from build123d import *

# Parameters (mm, degrees)
F0_R     = 10
F1_DEPTH = 25
F4_R     = 4
F5_DEPTH = 25


with BuildPart() as f1:
    # F0 (on Right) → F1 (new body)
    with BuildSketch(Plane.YZ):
        Circle(F0_R)
    extrude(amount=F1_DEPTH)


with BuildPart() as f2_1:
    # F2: copy of F1
    add(f1.part)

    # F4 (on face) → F5 (cut, through all)
    with BuildSketch(Plane.YZ.offset(25)):
        Circle(F4_R)
    extrude(amount=-F5_DEPTH, mode=Mode.SUBTRACT)


solid = f2_1.part
Part model, mm, in its own coordinate system. Round coordinates to 2 decimals unless told otherwise and drop trailing zeros. Write each loop counter-clockwise with the first axis right and the second up, starting at its lowest first coordinate (ties: lowest second). Pieces come first, ordered by that corner, then holes. Notation, with made-up numbers: M 20.25,74.25 L 61.25,74.25 A31 cw 61.25,100.25 Z; hole C 9,-17 d10. An arc over 180 degrees is marked long. Return JSON: item names as keys, results as strings. Group by question number.
(1) Saw through at D-D on x = 18. Write the cut outline in (y, z), then the cut area to 3 significant figures.
(2) Two-plate mould, pull along Z, no slides. Class faces 1 (the face through (0, -0.1, -4.3)), 2 (the face through (12.675, -0.867, -3.905)), 3 (the face through (12.32, -2.17, -9.76)): +Z half, -Z half, draft (parallel to the pull), parting line (faces both ways), or undercut.
(3) Drill centre lines: probe 1 along Z at (x, y) = (13.25, 0); probe 2 along Y at (x, z) = (22.25, 1.25); probe 3 along Z at (x, y) = (18.75, -1). Where is each one in solid material? Low to high.
(4) Pin check, flat tips, straight feed: pin 1 Ø7 at (y, z) = (0, 0) entering from +X; pin 2 Ø10 at (x, y) = (21, 6.5) entering from -Z; pin 3 Ø6 at (x, y) = (15, 8) entering from -Z. Stop position of each tip, or through.
(5) Saw through at A-A on z = 0. Write the cut outline in (x, y).
(6) Saw through at C-C on y = -8. Write the cut outline in (x, z), then the cut area to 3 significant figures.
Returned:
{
 "1": {"outline": "C 0,0 d20; hole C 0,0 d8", "area": "264 mm²"},
 "2": {"face 1": "draft", "face 2": "undercut", "face 3": "parting line"},
 "3": {"probe 1": "-10 to -4, 4 to 10", "probe 2": "-9.92 to -3.8, 3.8 to 9.92", "probe 3": "-9.95 to -3.87, 3.87 to 9.95"},
 "4": {"pin 1": "through", "pin 2": "z = -9.89", "pin 3": "z = -8.66"},
 "5": {"outline": "M 0,-10 L 25,-10 L 25,-4 L 0,-4 Z; M 0,4 L 25,4 L 25,10 L 0,10 Z"},
 "6": {"outline": "M 0,-6 L 25,-6 L 25,6 L 0,6 Z", "area": "300 mm²"}
}
